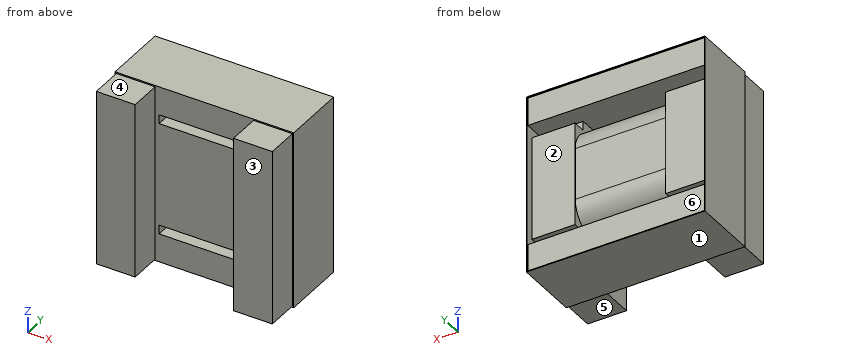
```python
from build123d import *

# Parameters (mm, degrees)
ESBO_O1_W                = 13.8
ESBO_O1_H                = 13.8
RESSALTO_EXTRUS_O1_DEPTH = 5
ESBO_O3_W                = 3
ESBO_O3_H                = 13.6
RESSALTO_EXTRUS_O3_DEPTH = 2.5
ESBO_O4_W                = 13.7
ESBO_O4_H                = 13.7
CORTE_EXTRUS_O1_DEPTH    = 0.1
ESBO_O5_W                = 13.7
ESBO_O5_H                = 9.4
CORTE_EXTRUS_O2_DEPTH    = 0.5
ESBO_O6_W                = 13.7
ESBO_O6_H                = 0.7
CORTE_EXTRUS_O3_DEPTH    = 1
ESBO_O7_W                = 7
ESBO_O7_H                = 0.7
CORTE_EXTRUS_O4_DEPTH    = 10
ESBO_O8_W                = 7
ESBO_O8_H                = 8
CORTE_EXTRUS_O5_DEPTH    = 0.02
FILETE1_R                = 2


with BuildPart() as part:
    # Esboço1 → Ressalto-extrusão1 (new body)
    with BuildSketch(Plane(origin=(0, 0, 0), x_dir=(1, 0, 0), z_dir=(0, 1, 0))):
        Rectangle(ESBO_O1_W, ESBO_O1_H)
    extrude(amount=RESSALTO_EXTRUS_O1_DEPTH)

    # Esboço3 → Ressalto-extrusão3 (add)
    with BuildSketch(Plane.XZ):
        with Locations((-5.3, 0)):
            Rectangle(ESBO_O3_W, ESBO_O3_H)
        with Locations((5.3, 0)):
            Rectangle(ESBO_O3_W, ESBO_O3_H)
    extrude(amount=RESSALTO_EXTRUS_O3_DEPTH)

    # Esboço4 → Corte-extrusão1 (cut)
    with BuildSketch(Plane(origin=(0, 5, 0), x_dir=(1, 0, 0), z_dir=(0, 1, 0))):
        Rectangle(ESBO_O4_W, ESBO_O4_H)
    extrude(amount=-CORTE_EXTRUS_O1_DEPTH, mode=Mode.SUBTRACT)

    # Esboço5 → Corte-extrusão2 (cut)
    with BuildSketch(Plane(origin=(0, 4.9, 0), x_dir=(1, 0, 0), z_dir=(0, 1, 0))):
        Rectangle(ESBO_O5_W, ESBO_O5_H)
    extrude(amount=-CORTE_EXTRUS_O2_DEPTH, mode=Mode.SUBTRACT)

    # Esboço6 → Corte-extrusão3 (cut)
    with BuildSketch(Plane(origin=(0, 4.4, 0), x_dir=(-1, 0, 0), z_dir=(0, 1, 0))):
        with Locations((0, -4.35)):
            Rectangle(ESBO_O6_W, ESBO_O6_H)
        with Locations((0, 4.35)):
            Rectangle(ESBO_O6_W, ESBO_O6_H)
    extrude(amount=-CORTE_EXTRUS_O3_DEPTH, mode=Mode.SUBTRACT)

    # Esboço7 → Corte-extrusão4 (cut)
    with BuildSketch(Plane(origin=(0, 3.4, 0), x_dir=(1, 0, 0), z_dir=(0, 1, 0))):
        with Locations((0, 4.35)):
            Rectangle(ESBO_O7_W, ESBO_O7_H)
        with Locations((0, -4.35)):
            Rectangle(ESBO_O7_W, ESBO_O7_H)
    extrude(amount=-CORTE_EXTRUS_O4_DEPTH, mode=Mode.SUBTRACT)

    # Esboço8 → Corte-extrusão5 (cut)
    with BuildSketch(Plane(origin=(0, 4.4, 0), x_dir=(1, 0, 0), z_dir=(0, 1, 0))):
        Rectangle(ESBO_O8_W, ESBO_O8_H)
    extrude(amount=-CORTE_EXTRUS_O5_DEPTH, mode=Mode.SUBTRACT)

    # Filete1
    # the kernel refuses this fillet: 2 mm, written as the material it takes off along each edge
    with BuildSketch(Plane(origin=(-3.5, 4.38, -4), x_dir=(0, -1, 0), z_dir=(1, 0, 0)), Plane(origin=(3.5, 4.38, 4), x_dir=(0, -1, 0), z_dir=(-1, 0, 0))) as filete1_piece_1:
        with BuildLine():
            CenterArc((FILETE1_R, -FILETE1_R), FILETE1_R, 90, 90)
            Line((0, -FILETE1_R), (0, 0))
            Line((0, 0), (FILETE1_R, 0))
        make_face()
    extrude(amount=7, mode=Mode.SUBTRACT)


solid = part.part
```
Geometry check sheet. Reference: the model listing, model coordinates, mm. Face numbers are marked on the shaded views. A direction names the side the tool comes from. Coordinates: 2 decimals unless noted, no trailing zeros. Write each loop counter-clockwise with the first axis right and the second up, starting at its lowest first coordinate (ties: lowest second). Pieces come first, ordered by that corner, then holes. Notation, with made-up numbers: M 26,77 L 62,77 A25 cw 62,91 Z; hole C 64,77 d10. An arc over 180 degrees is marked long. Answer as a JSON object with one key per item and string values.
1. Section check A-A, the plane y = 0.75. Enter the section's corners in (x, z), plus the area to 3 significant figures.
Answers below:
{"outline": "M -6.9,-6.9 L 6.9,-6.9 L 6.9,6.9 L -6.9,6.9 Z; hole M -3.5,-4.7 L 3.5,-4.7 L 3.5,-4 L -3.5,-4 Z; hole M -3.5,4 L 3.5,4 L 3.5,4.7 L -3.5,4.7 Z", "area": "181 mm²"}
2. Scan lines: L1, parallel to Z at x = -3, y = 1; L2, parallel to X at y = -2, z = -0.25; L3, parallel to Z at x = 6.5, y = 4.5. Record each from-to range of solid material in increasing order.
Answers below:
{"L1": "z = -6.9 to -4.7, -4 to 4, 4.7 to 6.9", "L2": "x = -6.8 to -3.8, 3.8 to 6.8", "L3": "z = -6.9 to -4.7, 4.7 to 6.9"}
3. Section check D-D, the plane x = 6. Enter the section's corners in (y, z), plus the area to 3 significant figures.
Answers below:
{"outline": "M -2.5,-6.8 L 0,-6.8 L 0,-6.9 L 5,-6.9 L 5,-6.85 L 4.9,-6.85 L 4.9,-4.7 L 3.4,-4.7 L 3.4,-4 L 4.4,-4 L 4.4,4 L 3.4,4 L 3.4,4.7 L 4.9,4.7 L 4.9,6.85 L 5,6.85 L 5,6.9 L 0,6.9 L 0,6.8 L -2.5,6.8 Z", "area": "95.5 mm²"}
4. Go/stop test with flat-tipped pins: pin 1 Ø3 at (x, z) = (-1.5, 1) entering from +Y; pin 2 Ø1.2 at (y, z) = (-1, -3.5) entering from -X; pin 3 Ø1.1 at (x, z) = (-0.5, -5.5) entering from +Y. Record where each tip stops, or that it passes through.
Answers below:
{"pin 1": "stops at y = 4.38", "pin 2": "stops at x = -6.8", "pin 3": "stops at y = 4.9"}
5. Section check B-B, the plane x = 0. Enter the section's corners in (y, z), plus the area to 3 significant figures.
Answers below:
{"outline": "M 0,-6.9 L 5,-6.9 L 5,-6.85 L 4.9,-6.85 L 4.9,-4.7 L 0,-4.7 Z; M 0,-4 L 2.38,-4 A2 ccw 4.38,-2 L 4.38,2 A2 ccw 2.38,4 L 0,4 Z; M 0,4.7 L 4.9,4.7 L 4.9,6.85 L 5,6.85 L 5,6.9 L 0,6.9 Z", "area": "54.9 mm²"}
6. Draft check along Z on the marked faces 1, 2 and 3. Enter one of: released by +Z, released by -Z, zero draft, split by the parting line, or undercut.
Answers below:
{"face 1": "released by -Z", "face 2": "undercut", "face 3": "zero draft"}
7. Tool access check on the marked faces 4, 5 and 6. Record the directions out of +Z, -Z, +X, -X, +Y, -Y that give a thin tool (end or side, any length) a straight path to the whole face; none if there is none.
Answers below:
{"face 4": "+Z, +X, -X, -Y", "face 5": "-Z, +X, -X, -Y", "face 6": "+Y"}
